Here's how the part is built. I have some questions about the finished solid (model axes, mm). A direction names the side the tool comes from. Round coordinates to 2 decimals unless told otherwise and drop trailing zeros. Order: outer loops, then holes, each group sorted by start corner. A loop starts at its lowest first (then second) coordinate and runs counter-clockwise, first axis right, second up. Notation, with made-up numbers: (76, 10) -> (89, 10) arc R15 ccw to (89, 37) -> close; hole circle Ø2 at (63.5, -23). An arc over 180 degrees is marked (long way). Use a Markdown table: item, result. Add a question column.
(1) On a 3-axis mill with a long thin cutter (end or side, diameter ignored), from which of +Z, -Z, +X, -X, +Y, -Y can I reach the whole of each face in a straight line? I mean faces 4 (the face through (75, 7, 40)), 5 (the face through (58.469, 2.535, 41.863)). Say none if no direction works.
(2) Thinking about a two-plate mould opening in X: for faces 1 (the face through (0, 5, 41)), 2 (the face through (39, 5, 80)), 3 (the face through (40, 5, 40)), which applies, pulls with the +X half, pulls with the -X half, needs draft (parallel to the pull), parting line crosses it, or undercut?
(3) I'm going to push a flat-ended pin straight in: P1, Ø6.5, axis at x = 22.5, z = 40, coming from the +Y side. Where does the tip first touch, or does it pass through?
(4) I want a section at C-C, the plane y = 8.75. Please give me the cut outline in (x, z).
(5) I want a section at D-D, the plane z = 16. Please give me the cut outline in (x, y), then the cut area to 3 significant figures.
(6) If I drill on probe 1 along X at (y, z) = (2.15, 40); probe 2 along X at (y, z) = (5.25, 38), over which ranges is the centre line in solid material (lowest first)?
(7) I want a section at B-B, the plane x = 57.5. Please give me the cut outline in (y, z), then the cut area to 3 significant figures.
(8) I want a section at A-A, the plane z = 40. Please give me the cut outline in (x, y), then the cut area to 3 significant figures.
from build123d import *

# Parameters (mm, degrees)
SKETCH1_W           = 80
SKETCH1_H           = 80
BOSS_EXTRUDE1_DEPTH = 5
SKETCH2_W           = 80
SKETCH2_H           = 80
SKETCH2_W_2         = 70
SKETCH2_H_2         = 70
BOSS_EXTRUDE2_DEPTH = 5
CUT_EXTRUDE1_REACH  = 7
SKETCH3_R           = 2.1


with BuildPart() as part:
    # Sketch1 → Boss-Extrude1 (new body)
    with BuildSketch(Plane(origin=(0, 0, 0), x_dir=(1, 0, 0), z_dir=(0, 1, 0))):
        with Locations((40, -40)):
            Rectangle(SKETCH1_W, SKETCH1_H)
    extrude(amount=BOSS_EXTRUDE1_DEPTH)

    # Sketch2 → Boss-Extrude2 (add)
    with BuildSketch(Plane(origin=(0, 5, 0), x_dir=(1, 0, 0), z_dir=(0, 1, 0))):
        with Locations((40, -40)):
            Rectangle(SKETCH2_W, SKETCH2_H)
        with Locations((40, -40)):
            Rectangle(SKETCH2_W_2, SKETCH2_H_2, mode=Mode.SUBTRACT)
    extrude(amount=BOSS_EXTRUDE2_DEPTH)

    # Sketch3 → Cut-Extrude1 (cut, up to next)
    with BuildSketch(Plane(origin=(0, 5, 0), x_dir=(1, 0, 0), z_dir=(0, 1, 0)), mode=Mode.PRIVATE) as cut_extrude1_sk1:
        with Locations((22.5, -40)):
            Circle(SKETCH3_R)
    cut_extrude1_tool1 = extrude(cut_extrude1_sk1.sketch, amount=-CUT_EXTRUDE1_REACH, mode=Mode.PRIVATE) & part.part
    add(cut_extrude1_tool1.solids().sort_by_distance((22.5, 5, 40))[0], mode=Mode.SUBTRACT)
    # Sketch3 → Cut-Extrude1 (cut, up to next)
    with BuildSketch(Plane(origin=(0, 5, 0), x_dir=(1, 0, 0), z_dir=(0, 1, 0)), mode=Mode.PRIVATE) as cut_extrude1_sk2:
        with Locations((57.5, -40)):
            Circle(SKETCH3_R)
    cut_extrude1_tool2 = extrude(cut_extrude1_sk2.sketch, amount=-CUT_EXTRUDE1_REACH, mode=Mode.PRIVATE) & part.part
    add(cut_extrude1_tool2.solids().sort_by_distance((57.5, 5, 40))[0], mode=Mode.SUBTRACT)


solid = part.part
Taken from the geometry:
| question | item | result |
|---|---|---|
| 1 | face 4 | +Y |
| 1 | face 5 | +Y, -Y |
| 2 | face 1 | pulls with the -X half |
| 2 | face 2 | needs draft |
| 2 | face 3 | undercut |
| 3 | P1 | stops at y = 5 |
| 4 | outline | (0, 0) -> (80, 0) -> (80, 80) -> (0, 80) -> close; hole (5, 5) -> (75, 5) -> (75, 75) -> (5, 75) -> close |
| 5 | outline | (0, 0) -> (80, 0) -> (80, 10) -> (75, 10) -> (75, 5) -> (5, 5) -> (5, 10) -> (0, 10) -> close |
| 5 | area | 450 mm2 |
| 6 | probe 1 | x = 0 to 20.4, 24.6 to 55.4, 59.6 to 80 |
| 6 | probe 2 | x = 0 to 5, 75 to 80 |
| 7 | outline | (0, 0) -> (10, 0) -> (10, 5) -> (5, 5) -> (5, 37.9) -> (0, 37.9) -> close; (0, 42.1) -> (5, 42.1) -> (5, 75) -> (10, 75) -> (10, 80) -> (0, 80) -> close |
| 7 | area | 429 mm2 |
| 8 | outline | (0, 0) -> (20.4, 0) -> (20.4, 5) -> (5, 5) -> (5, 10) -> (0, 10) -> close; (24.6, 0) -> (55.4, 0) -> (55.4, 5) -> (24.6, 5) -> close; (59.6, 0) -> (80, 0) -> (80, 10) -> (75, 10) -> (75, 5) -> (59.6, 5) -> close |
| 8 | area | 408 mm2 |
